Could you check a few things on this model? Use its own coordinates, in mm. A direction names the side the tool comes from. Give positions to 0.01 mm unless a question says otherwise; leave off trailing zeros. Loops run counter-clockwise (first coordinate to the right, second up) from the corner with the lowest first, then second, coordinate; pieces in that order, holes last. Notation, with made-up numbers: (-30.75, 14.5) - (-17.75, 14.5) arc R31 cw to (-17.75, 52.5) - close; hole circle Ø11 at (62, 52.25). An arc over 180 degrees is marked (long way). Answer in a Markdown table with one row per item. Add a question column.
```python
from build123d import *

# Parameters (mm, degrees)
FILLET1_R               = 0.3
SKETCH3_R               = 3.6
CUT_EXTRUDE1_DEPTH      = 1
CUT_EXTRUDE1_DEPTH_BACK = 22
FILLET2_R               = 0.5
FILLET3_R               = 0.5
SKETCH5_W               = 6.5
SKETCH5_H               = 2
SKETCH6_W               = 8.5
SKETCH6_H               = 2
SKETCH8_W               = 8.5
SKETCH8_H               = 3
SKETCH7_W               = 6.5
SKETCH7_H               = 3
SKETCH11_R              = 5.52
CUT_EXTRUDE3_DEPTH      = 10
CUT_EXTRUDE4_DEPTH      = 10
BOSS_EXTRUDE1_DEPTH     = 3
SKETCH15_R              = 23
SKETCH15_R_2            = 8.340902118
SKETCH15_R_3            = 5.6
BOSS_EXTRUDE4_DEPTH     = 3
SKETCH16_R              = 5.52
CUT_EXTRUDE6_DEPTH      = 3


with BuildPart() as part:
    # Sketch2 → Revolve1 (revolve)
    with BuildSketch(Plane.XY):
        Polygon((2, 0), (2.6, 0), (8.340902118, -16), (20.340902118, -16), (20.340902118, -19), (6.4, -19), (6.4, -37.427752697), (3.4, -37.427752697), (3.4, -16), (2, -16), align=None)
    revolve(axis=Axis((0, 0, 0), (0, -1, 0)))

    # Fillet1
    fillet1_edges = [part.edges().sort_by_distance(p)[0] for p in [
        (-2, 0, 0),
    ]]
    fillet(fillet1_edges, radius=FILLET1_R)

    # Sketch3 → Cut-Extrude1 (cut, two sides)
    with BuildSketch(Plane.XZ.offset(37.427752697)) as cut_extrude1_sk:
        Circle(SKETCH3_R)
    extrude(amount=CUT_EXTRUDE1_DEPTH, mode=Mode.SUBTRACT)
    extrude(cut_extrude1_sk.sketch, amount=-CUT_EXTRUDE1_DEPTH_BACK, mode=Mode.SUBTRACT)

    # Fillet2
    fillet2_edges = [part.edges().sort_by_distance(p)[0] for p in [
        (-2, -15.427752697, 0),
    ]]
    fillet(fillet2_edges, radius=FILLET2_R)

    # Fillet3
    fillet3_edges = [part.edges().sort_by_distance(p)[0] for p in [
        (-3.6, -37.427752697, 0),
    ]]
    fillet(fillet3_edges, radius=FILLET3_R)

    # Sketch5 → Cut-Loft2 section 0
    with BuildSketch(Plane(origin=(0, -16, 0), x_dir=(1, 0, 0), z_dir=(0, 1, 0))):
        with Locations((0, -15)):
            Rectangle(SKETCH5_W, SKETCH5_H)
    # Sketch6 → Cut-Loft2 section 1
    with BuildSketch(Plane.XZ.offset(19)):
        with Locations((0, 15)):
            Rectangle(SKETCH6_W, SKETCH6_H)
    loft(mode=Mode.SUBTRACT)

    # Sketch8 → Cut-Loft3 section 0
    with BuildSketch(Plane.XZ.offset(19)):
        with Locations((0, 15)):
            Rectangle(SKETCH8_W, SKETCH8_H)
    # Sketch7 → Cut-Loft3 section 1
    with BuildSketch(Plane(origin=(0, -16, 0), x_dir=(1, 0, 0), z_dir=(0, 1, 0))):
        with Locations((0, -15)):
            Rectangle(SKETCH7_W, SKETCH7_H)
    loft(mode=Mode.SUBTRACT)

    # Sketch11 → Cut-Extrude3 (cut)
    with BuildSketch(Plane(origin=(0, -16, 0), x_dir=(1, 0, 0), z_dir=(0, 1, 0))):
        with Locations((0, 14.340902118)):
            Circle(SKETCH11_R)
        with Locations((12.419585547, 7.170451059)):
            Circle(SKETCH11_R)
        with BuildLine():
            ThreePointArc((-17.200045776, 9.930451059), (-15.179585547, 2.38999083), (-7.639125318, 4.410451059))
            Line((-7.639125318, 4.410451059), (-12.419585547, 7.170451059))
            Line((-12.419585547, 7.170451059), (-17.200045776, 9.930451059))
        make_face()
        with BuildLine():
            Line((-12.419585547, 7.170451059), (-7.639125318, 4.410451059))
            ThreePointArc((-7.639125318, 4.410451059), (-7.087674986, 5.74176993), (-6.899585547, 7.170451059))
            ThreePointArc((-6.899585547, 7.170451059), (-10.990904418, 12.50236162), (-17.200045776, 9.930451059))
            Line((-17.200045776, 9.930451059), (-12.419585547, 7.170451059))
        make_face()
    extrude(amount=-CUT_EXTRUDE3_DEPTH, mode=Mode.SUBTRACT)

    # Sketch13 → Cut-Extrude4 (cut)
    with BuildSketch(Plane(origin=(0, -16, 0), x_dir=(1, 0, 0), z_dir=(0, 1, 0))):
        with BuildLine():
            Line((-8.340902118, 0), (-20.340902118, 0))
            ThreePointArc((-20.340902118, 0), (-17.61573797, -10.170451059), (-10.170451059, -17.61573797))
            Line((-10.170451059, -17.61573797), (-4.170451059, -7.223433125))
            ThreePointArc((-4.170451059, -7.223433125), (-7.223433125, -4.170451059), (-8.340902118, 0))
        make_face()
        with BuildLine():
            Line((8.340902118, 0), (20.340902118, 0))
            ThreePointArc((20.340902118, 0), (17.546873261, -10.288806428), (9.932362997, -17.751069384))
            Line((9.932362997, -17.751069384), (4.072821701, -7.278926537))
            ThreePointArc((4.072821701, -7.278926537), (7.195194761, -4.218983349), (8.340902118, 0))
        make_face()
    extrude(amount=-CUT_EXTRUDE4_DEPTH, mode=Mode.SUBTRACT)

    # Sketch14 → Boss-Extrude1 (add)
    with BuildSketch(Plane(origin=(0, -16, 0), x_dir=(1, 0, 0), z_dir=(0, 1, 0))):
        with BuildLine():
            ThreePointArc((0, 20.340902118), (14.383189823, 14.383189823), (20.340902118, 0))
            Line((20.340902118, 0), (23, 0))
            ThreePointArc((23, 0), (16.263455967, 16.263455967), (0, 23))
            Line((0, 23), (0, 20.340902118))
        make_face()
        with BuildLine():
            Line((-23, 0), (-20.340902118, 0))
            ThreePointArc((-20.340902118, 0), (-14.383189823, 14.383189823), (0, 20.340902118))
            Line((0, 20.340902118), (0, 23))
            ThreePointArc((0, 23), (-16.263455967, 16.263455967), (-23, 0))
        make_face()
    extrude(amount=-BOSS_EXTRUDE1_DEPTH)

    # Sketch15 → Boss-Extrude4 (add)
    with BuildSketch(Plane(origin=(0, -16, 0), x_dir=(1, 0, 0), z_dir=(0, 1, 0))):
        Circle(SKETCH15_R)
        Circle(SKETCH15_R_2, mode=Mode.SUBTRACT)
        with Locations((-12.419585547, 7.170451059)):
            Circle(SKETCH15_R_3, mode=Mode.SUBTRACT)
        with Locations((12.419585547, 7.170451059)):
            Circle(SKETCH15_R_3, mode=Mode.SUBTRACT)
        with Locations((0, -14.340902118)):
            Circle(SKETCH15_R_3, mode=Mode.SUBTRACT)
    extrude(amount=-BOSS_EXTRUDE4_DEPTH)

    # Sketch16 → Cut-Extrude6 (cut)
    with BuildSketch(Plane(origin=(0, -16, 0), x_dir=(1, 0, 0), z_dir=(0, 1, 0))):
        with Locations((0, -14.34090212)):
            Circle(SKETCH16_R)
    extrude(amount=-CUT_EXTRUDE6_DEPTH, mode=Mode.SUBTRACT)


solid = part.part
```
(1) I want a section at B-B on z = 19. Please give me the cut outline in (x, y), then the cut area to 3 significant figures.
(2) I want a section at A-A on x = -11. Please give me the cut outline in (y, z), then the cut area to 3 significant figures.
(3) Please list where these lines run through material, in increasing order: line 1 (Z direction, x = 0, y = -17); line 2 (Z direction, x = 0, y = -27.25); line 3 (Y direction, x = -19, z = 10.5).
(4) I want a section at C-C on y = -21.5. Please give me the cut outline in (x, z).
(5) I want a section at D-D on z = -17.5. Please give me the cut outline in (x, y).
(6) For pin 1 Ø1.5 at (x, z) = (-12, -10) entering from -Y; pin 2 Ø12 at (x, z) = (13.5, 10.5) entering from +Y; pin 3 Ø14.5 at (x, z) = (12.42, -7.17) entering from -Y; pin 4 Ø1 at (y, z) = (-12.5, 3.5) entering from +X, each with a flat end and sliding along its axis, tell me the tip position at first contact or that it passes through.
(7) We'd pull the mould along Z, two halves only. Please class faces 3 (the flat face through (-0.9, -15.428, 2.5)), 4 (the conical face through (-0.63, -6.33, 4.83)), 5 (the flat face through (4.2, -37.428, -1.3)): pulls with the +Z half, pulls with the -Z half, needs draft (parallel to the pull), parting line crosses it, or undercut.
(8) On a 3-axis mill with a long thin cutter (end or side, diameter ignored), from which of +Z, -Z, +X, -X, +Y, -Y can I reach the whole of each face in a straight line? I mean faces 1 (the cylindrical face through (-5.08, -28.34, -3.89)), 2 (the cylindrical face through (17.685, -17.479, -8.829)). Say none if no direction works.
Reported:
| question | item | result |
|---|---|---|
| 1 | outline | (-12.96, -19) - (-2.96, -19) - (-2.96, -16) - (-12.96, -16) - close; (2.96, -19) - (12.96, -19) - (12.96, -16) - (2.96, -16) - close |
| 1 | area | 60.0 mm² |
| 2 | outline | (-19, -20.2) - (-16, -20.2) - (-16, -12.5) - (-19, -12.5) - close; (-19, -1.84) - (-16, -1.84) - (-16, 20.2) - (-19, 20.2) - close |
| 2 | area | 89.2 mm² |
| 3 | line 1 | -23 to -3.6, 3.6 to 8.82, 19.86 to 23 |
| 3 | line 2 | -6.4 to -3.6, 3.6 to 6.4 |
| 3 | line 3 | -19 to -16 |
| 4 | outline | circle Ø12.8 at (0, 0); hole circle Ø7.2 at (0, 0) |
| 5 | outline | (-14.92, -19) - (14.92, -19) - (14.92, -16) - (-14.92, -16) - close |
| 6 | pin 1 | through |
| 6 | pin 2 | y = -16 |
| 6 | pin 3 | y = -19 |
| 6 | pin 4 | x = 6.49 |
| 7 | face 3 | undercut |
| 7 | face 4 | parting line crosses it |
| 7 | face 5 | needs draft |
| 8 | face 1 | -Y |
| 8 | face 2 | +Y, -Y |
